For this review, take the finished solid that the model builds, in its own axes (mm). A direction names the side the tool comes from. Give positions to 0.01 mm unless a question says otherwise; leave off trailing zeros. Write each loop counter-clockwise with the first axis right and the second up, starting at its lowest first coordinate (ties: lowest second). Pieces come first, ordered by that corner, then holes. Notation, with made-up numbers: (28.5, 57) -> (74.5, 57) arc R19 cw to (74.5, 82) -> close; hole circle Ø4 at (58.5, 9.25). An arc over 180 degrees is marked (long way). Write item = value, one per line.
```python
from build123d import *

# Parameters (mm, degrees)
SKETCH1_W             = 25
SKETCH1_H             = 25
SKETCH1_W_2           = 20
SKETCH1_H_2           = 20
BOSS_EXTRUDE1_DEPTH   = 500
SKETCH2_W             = 125
SKETCH2_H             = 125
SKETCH2_W_2           = 25
SKETCH2_H_2           = 25
BOSS_EXTRUDE2_DEPTH   = 7.5
F_3_0MM_DOWEL_HOLE1_D = 3
SKETCH7_W             = 25
SKETCH7_H             = 25
SKETCH7_W_2           = 20
SKETCH7_H_2           = 20
BOSS_EXTRUDE3_DEPTH   = 400
SKETCH8_W             = 25
SKETCH8_H             = 25
SKETCH8_W_2           = 20
SKETCH8_H_2           = 20
BOSS_EXTRUDE4_DEPTH   = 400


with BuildPart() as part:
    # Sketch1 → Boss-Extrude1 (new body)
    with BuildSketch(Plane(origin=(0, 0, 0), x_dir=(1, 0, 0), z_dir=(0, 1, 0))):
        with Locations((12.5, 12.5)):
            Rectangle(SKETCH1_W, SKETCH1_H)
        with Locations((12.5, 12.5)):
            Rectangle(SKETCH1_W_2, SKETCH1_H_2, mode=Mode.SUBTRACT)
    extrude(amount=BOSS_EXTRUDE1_DEPTH)

    # Sketch2 → Boss-Extrude2 (add)
    with BuildSketch(Plane(origin=(0, 500, 0), x_dir=(1, 0, 0), z_dir=(0, 1, 0))):
        with Locations((12.5, 12.5)):
            Rectangle(SKETCH2_W, SKETCH2_H)
        with Locations((12.5, 12.5)):
            Rectangle(SKETCH2_W_2, SKETCH2_H_2, mode=Mode.SUBTRACT)
    extrude(amount=-BOSS_EXTRUDE2_DEPTH)

    # Ø3.0mm Dowel Hole1 (through all)
    with Locations(Plane(origin=(0, 500, 0), x_dir=(1, 0, 0), z_dir=(0, 1, 0))):
        with Locations((-35, 60), (12.5, 60), (60, 60), (60, 12.5), (60, -35), (12.5, -35), (-35, -35), (-35, 12.5), (12.5, 45), (12.5, -20), (-11.25, 45), (36.25, 45), (-11.25, -20), (36.25, -20)):
            Hole(F_3_0MM_DOWEL_HOLE1_D / 2)

    # Sketch7 → Boss-Extrude3 (add)
    with BuildSketch(Plane(origin=(0, 0, -25), x_dir=(-1, 0, 0), z_dir=(0, 0, -1))):
        with Locations((-12.5, 12.5)):
            Rectangle(SKETCH7_W, SKETCH7_H)
        with Locations((-12.5, 12.5)):
            Rectangle(SKETCH7_W_2, SKETCH7_H_2, mode=Mode.SUBTRACT)
    extrude(amount=BOSS_EXTRUDE3_DEPTH)

    # Sketch8 → Boss-Extrude4 (add)
    with BuildSketch(Plane(origin=(25, 0, 0), x_dir=(0, 0, -1), z_dir=(1, 0, 0))):
        with Locations((12.5, 12.5)):
            Rectangle(SKETCH8_W, SKETCH8_H)
        with Locations((12.5, 12.5)):
            Rectangle(SKETCH8_W_2, SKETCH8_H_2, mode=Mode.SUBTRACT)
    extrude(amount=BOSS_EXTRUDE4_DEPTH)


solid = part.part
```
(1) To check wall thickness, follow probe 1 along Z at (x, y) = (60, 496); probe 2 along Z at (x, y) = (12.5, 495.5); probe 3 along X at (y, z) = (497.5, -45). State the ranges of each line that lie inside material, in increasing order.
Answers below:
probe_1 = -75 to -61.5, -58.5 to -14, -11 to 33.5, 36.5 to 50
probe_2 = -75 to -61.5, -58.5 to -46.5, -43.5 to -22.5, -2.5 to 18.5, 21.5 to 33.5, 36.5 to 50
probe_3 = -50 to -12.75, -9.75 to 11, 14 to 34.75, 37.75 to 75
(2) The part is to be moulded in two halves that separate along X. For faces 1 (the face through (12, 12, -25)), 2 (the face through (425, 13, -23)), 3 (the face through (12, 255, -25)), say which applies: released by +X, released by -X, zero draft, split by the parting line, or undercut.
Answers below:
face_1 = undercut
face_2 = released by +X
face_3 = zero draft
(3) Tool access review of faces 4 (the face through (222, 12, -22.5)), 5 (the face through (13, 2.5, -222)), 6 (the face through (22.5, 246, -12)), 7 (the face through (23, 172, 0)): name each direction out of +Z, -Z, +X, -X, +Y, -Y from which nothing blocks a thin tool from reaching the whole face with its end or side.
Answers below:
face_4 = +X
face_5 = -Z
face_6 = +Y, -Y
face_7 = +Z, +X, -X, -Y
(4) Take a section at B-B (z = -339.5). Write out the cut boundary in (x, y).
Answers below:
outline = (0, 0) -> (25, 0) -> (25, 25) -> (0, 25) -> close; hole (2.5, 2.5) -> (22.5, 2.5) -> (22.5, 22.5) -> (2.5, 22.5) -> close
(5) Take a section at A-A (y = 116). Write out the cut boundary in (x, z), plus the area to 3 significant figures.
Answers below:
outline = (0, -25) -> (25, -25) -> (25, 0) -> (0, 0) -> close; hole (2.5, -22.5) -> (22.5, -22.5) -> (22.5, -2.5) -> (2.5, -2.5) -> close
area = 225 mm^2
(6) For pin 1 (8 mm diameter, centred on y = 498, z = -35.5, fed in from +X); pin 2 (3 mm diameter, centred on x = 229.5, z = -24, fed in from +Y); pin 3 (6 mm diameter, centred on y = 312.5, z = -9.5, fed in from +X); pin 4 (3.5 mm diameter, centred on x = 12.5, z = -45, fed in from -Y), all flat-tipped, find the tip position at first contact; note any pin that passes through.
Answers below:
pin_1 = 75
pin_2 = 25
pin_3 = 25
pin_4 = 0
